For this review, take the finished solid that the model builds, in its own axes (mm). A direction names the side the tool comes from. Give positions to 0.01 mm unless a question says otherwise; leave off trailing zeros. Order: outer loops, then holes, each group sorted by start corner. A loop starts at its lowest first (then second) coordinate and runs counter-clockwise, first axis right, second up.
Item 1: For P1, Ø2.5, axis at x = 52.56, z = -3.38, coming from the +Y side, flat-tipped, find the tip position at first contact; note if it passes through.
Item 2: Consider section B-B (x = 41.5). Give the boundary of the cut face in (y, z).
Item 3: Machinability: for faces 4 (the flat face through (29, 0.8, 1)), 5 (the flat face through (70.5, 2, 37)), 6 (the flat face through (77, 2, 50)), which of the approach directions +Z, -Z, +X, -X, +Y, -Y give a long, thin tool a straight path to every point of the face, cutting with its end or side? Answer none if there is none.
Item 4: The part is to be moulded in two halves that separate along Z. For faces 1 (the flat face through (77, 2, -50)), 2 (the flat face through (55, 2, 63)), 3 (the flat face through (94.5, 2, 37)), say which applies: released by +Z, released by -Z, zero draft, split by the parting line, or undercut.
Item 5: Consider section A-A (z = -38.5). Give the boundary of the cut face in (x, y), plus the area to 3 significant figures.
Item 6: Consider section C-C (y = 2.85). Give the number of separate pieces and of enclosed holes in the cut face, plus the area to 3 significant figures.
Item 7: For probe 1 along X at (y, z) = (1.3, -45); probe 2 along Z at (x, y) = (9, 2.45); probe 3 along X at (y, z) = (1.2, -22.5), list the stretches that pass through material, from the lowest coordinate up.
Item 8: Consider section D-D (x = 82.5). Give the boundary of the cut face in (y, z), plus the area to 3 significant figures.
```python
from build123d import *

# Parameters (mm, degrees)
SKETCH_1_W             = 200
SKETCH_1_H             = 150
EXTRUDE_1196_DEPTH     = 4
SKETCH_1250_R          = 1.5
SKETCH_1250_W          = 12.7
SKETCH_1250_H          = 5.08
SKETCH_1250_W_2        = 5.08
SKETCH_1250_H_2        = 22.86
SKETCH_1250_W_3        = 7.874
SKETCH_1250_H_3        = 6.858
DMOTOR_DEPTH           = 3.2
DMOTOR_2_OUTLINE_R     = 1.5
DMOTOR_2_OUTLINE_W     = 7.874
DMOTOR_2_OUTLINE_H     = 6.858
DMOTOR_2_OUTLINE_W_2   = 12.7
DMOTOR_2_OUTLINE_H_2   = 5.08
DMOTOR_2_OUTLINE_W_3   = 5.08
DMOTOR_2_OUTLINE_H_3   = 22.86
DMOTOR_2_DEPTH         = 4
LINELANCE_2_R          = 1.5
LINELANCE_2_W          = 2.54
LINELANCE_2_H          = 15.24
LINELANCE_DEPTH        = 126.063983624
SKETCH_3356_R          = 1.5
SKETCH_3356_W          = 45
SKETCH_3356_H          = 25
CUT_EXTRUDE_4137_DEPTH = 126.063983624


# Read off the part's stored shape, not the designer's step: Вырез для компонентов DMotor
with BuildPart() as part:
    # Эскиз1 → Extrude 1196 (new body)
    with BuildSketch(Plane(origin=(0, 0, 0), x_dir=(1, 0, 0), z_dir=(0, 1, 0))):
        Rectangle(SKETCH_1_W, SKETCH_1_H)
    extrude(amount=EXTRUDE_1196_DEPTH)

    # Sketch 1250 → DMotor (cut)
    with BuildSketch(Plane(origin=(0, 4, 0), x_dir=(1, 0, 0), z_dir=(0, 1, 0))):
        with BuildLine():
            Line((30.543559349, 14.375593505), (6.059123786, 14.375593505))
            ThreePointArc((6.059123786, 14.375593505), (4.291356833, 13.643360458), (3.559123786, 11.875593505))
            Line((3.559123786, 11.875593505), (3.559123786, -15.124406495))
            ThreePointArc((3.559123786, -15.124406495), (4.291356833, -16.892173448), (6.059123786, -17.624406495))
            Line((6.059123786, -17.624406495), (20.543559349, -17.624406495))
            ThreePointArc((20.543559349, -17.624406495), (22.559123786, -18.874406495), (24.574688223, -17.624406495))
            Line((24.574688223, -17.624406495), (53.059123786, -17.624406495))
            ThreePointArc((53.059123786, -17.624406495), (54.826890739, -16.892173448), (55.559123786, -15.124406495))
            Line((55.559123786, -15.124406495), (55.559123786, 11.875593505))
            ThreePointArc((55.559123786, 11.875593505), (54.826890739, 13.643360458), (53.059123786, 14.375593505))
            Line((53.059123786, 14.375593505), (34.574688223, 14.375593505))
            ThreePointArc((34.574688223, 14.375593505), (32.559123786, 15.625593505), (30.543559349, 14.375593505))
        make_face()
        with Locations(Location((22.559123786, -16.624406495, 0), (0, 0, 270))):
            Circle(SKETCH_1250_R, mode=Mode.SUBTRACT)
        with Locations(Location((32.559123786, 13.375593505, 0), (0, 0, 270))):
            Circle(SKETCH_1250_R, mode=Mode.SUBTRACT)
        with Locations(Location((52.559123786, 3.375593505, 0), (0, 0, 270))):
            Circle(SKETCH_1250_R, mode=Mode.SUBTRACT)
        with Locations((10.734123786, 10.235593505)):
            Rectangle(SKETCH_1250_W, SKETCH_1250_H, mode=Mode.SUBTRACT)
        with Locations((6.924123786, -4.509406495)):
            Rectangle(SKETCH_1250_W_2, SKETCH_1250_H_2, mode=Mode.SUBTRACT)
        with Locations((50.191123786, 8.914593505)):
            Rectangle(SKETCH_1250_W_3, SKETCH_1250_H_3, mode=Mode.SUBTRACT)
        with Locations((50.191123786, -12.163406495)):
            Rectangle(SKETCH_1250_W_3, SKETCH_1250_H_3, mode=Mode.SUBTRACT)
    extrude(amount=-DMOTOR_DEPTH, mode=Mode.SUBTRACT)

    # DMotor 2 outline → DMotor 2 (cut)
    with BuildSketch(Plane(origin=(0, 0, 0), x_dir=(1, 0, 0), z_dir=(0, 1, 0))):
        with Locations((32.559123786, 13.375593505)):
            Circle(DMOTOR_2_OUTLINE_R)
        with Locations((50.191123786, -12.163406495)):
            Rectangle(DMOTOR_2_OUTLINE_W, DMOTOR_2_OUTLINE_H)
        with Locations((50.191123786, 8.914593505)):
            Rectangle(DMOTOR_2_OUTLINE_W, DMOTOR_2_OUTLINE_H)
        with Locations((10.734123786, 10.235593505)):
            Rectangle(DMOTOR_2_OUTLINE_W_2, DMOTOR_2_OUTLINE_H_2)
        with Locations((6.924123786, -4.509406495)):
            Rectangle(DMOTOR_2_OUTLINE_W_3, DMOTOR_2_OUTLINE_H_3)
        with Locations((22.559123786, -16.624406495)):
            Circle(DMOTOR_2_OUTLINE_R)
        with Locations((52.559123786, 3.375593505)):
            Circle(DMOTOR_2_OUTLINE_R)
    extrude(amount=DMOTOR_2_DEPTH, mode=Mode.SUBTRACT)

    # Linelance 2 → Linelance (cut, through all)
    with BuildSketch(Plane(origin=(0, 4, 0), x_dir=(1, 0, 0), z_dir=(0, 1, 0))):
        with Locations(Location((-86.5, 22.5, 0), (0, 0, 270))):
            Circle(LINELANCE_2_R)
        with Locations(Location((-86.5, -22.5, 0), (0, 0, 270))):
            Circle(LINELANCE_2_R)
        with Locations((-84.03, 8.955)):
            Rectangle(LINELANCE_2_W, LINELANCE_2_H)
    extrude(amount=-LINELANCE_DEPTH, mode=Mode.SUBTRACT)

    # Sketch 3356 → Cut-Extrude 4137 (cut, through all)
    with BuildSketch(Plane(origin=(0, 4, 0), x_dir=(1, 0, 0), z_dir=(0, 1, 0))):
        with Locations(Location((72, 45, 0), (0, 0, 270))):
            Circle(SKETCH_3356_R)
        with Locations(Location((72, 29, 0), (0, 0, 270))):
            Circle(SKETCH_3356_R)
        with Locations(Location((96, 45, 0), (0, 0, 270))):
            Circle(SKETCH_3356_R)
        with Locations(Location((96, 29, 0), (0, 0, 270))):
            Circle(SKETCH_3356_R)
        with Locations(Location((96, -29, 0), (0, 0, 90))):
            Circle(SKETCH_3356_R)
        with Locations(Location((96, -45, 0), (0, 0, 90))):
            Circle(SKETCH_3356_R)
        with Locations(Location((72, -29, 0), (0, 0, 90))):
            Circle(SKETCH_3356_R)
        with Locations(Location((72, -45, 0), (0, 0, 90))):
            Circle(SKETCH_3356_R)
        with Locations((77.5, 62.5)):
            Rectangle(SKETCH_3356_W, SKETCH_3356_H)
        with Locations((77.5, -62.5)):
            Rectangle(SKETCH_3356_W, SKETCH_3356_H)
        with BuildLine():
            Line((73.5, 41), (73.5, 33))
            ThreePointArc((73.5, 33), (72, 31.5), (70.5, 33))
            Line((70.5, 33), (70.5, 41))
            ThreePointArc((70.5, 41), (72, 42.5), (73.5, 41))
        make_face()
        with BuildLine():
            Line((97.5, 41), (97.5, 33))
            ThreePointArc((97.5, 33), (96, 31.5), (94.5, 33))
            Line((94.5, 33), (94.5, 41))
            ThreePointArc((94.5, 41), (96, 42.5), (97.5, 41))
        make_face()
        with BuildLine():
            Line((73.5, -41), (73.5, -33))
            ThreePointArc((73.5, -33), (72, -31.5), (70.5, -33))
            Line((70.5, -33), (70.5, -41))
            ThreePointArc((70.5, -41), (72, -42.5), (73.5, -41))
        make_face()
        with BuildLine():
            Line((97.5, -41), (97.5, -33))
            ThreePointArc((97.5, -33), (96, -31.5), (94.5, -33))
            Line((94.5, -33), (94.5, -41))
            ThreePointArc((94.5, -41), (96, -42.5), (97.5, -41))
        make_face()
    extrude(amount=-CUT_EXTRUDE_4137_DEPTH, mode=Mode.SUBTRACT)


solid = part.part
```
Resolved:
1. P1: passes through
2. outline: (0, -75) - (4, -75) - (4, -14.38) - (0.8, -14.38) - (0.8, 17.62) - (4, 17.62) - (4, 75) - (0, 75) - close
3. face 4: +Y
3. face 5: +Y, -Y
3. face 6: +Z, +X, +Y, -Y
4. face 1: released by -Z
4. face 2: zero draft
4. face 3: undercut
5. outline: (-100, 0) - (70.5, 0) - (70.5, 4) - (-100, 4) - close; (73.5, 0) - (94.5, 0) - (94.5, 4) - (73.5, 4) - close; (97.5, 0) - (100, 0) - (100, 4) - (97.5, 4) - close
5. area: 776 mm2
6. separate pieces: 1
6. enclosed holes: 16
6. area: 25,900 mm2
7. probe 1: x = -100 to 70.5, 73.5 to 94.5, 97.5 to 100
7. probe 2: z = -75 to -14.38, 17.62 to 75
7. probe 3: x = -100 to -88, -85 to 100
8. outline: (0, -50) - (4, -50) - (4, 50) - (0, 50) - close
8. area: 400 mm2
